from build123d import *

# Parameters (mm, degrees)
F1_W          = 508
F1_H          = 254
F2_DEPTH      = 63.5
F4_R          = 38.1
F5_DEPTH      = 127
F5_DEPTH_BACK = 127
F6_R          = 57.15
F7_DEPTH      = 127
F7_DEPTH_BACK = 127
F3_R          = 19.05
F8_DEPTH      = 127
F9_SIZE2      = 12.7
F9_SIZE       = 12.7


with BuildPart() as f2:
    # F1 (on face) → F2 (new body)
    with BuildSketch(Plane.XY):
        with Locations((0, -127)):
            Rectangle(F1_W, F1_H)
    extrude(amount=F2_DEPTH)

    # F4 (on face) → F5 (cut, two sides)
    with BuildSketch(Plane.XY.offset(63.5)) as f5_sk:
        with Locations((-63.5, -127)):
            Circle(F4_R)
    extrude(amount=F5_DEPTH, mode=Mode.SUBTRACT)
    extrude(f5_sk.sketch, amount=-F5_DEPTH_BACK, mode=Mode.SUBTRACT)

    # F6 (on face) → F7 (cut, two sides)
    with BuildSketch(Plane.XY.offset(63.5)) as f7_sk:
        with Locations((127, -127)):
            Circle(F6_R)
    extrude(amount=F7_DEPTH, mode=Mode.SUBTRACT)
    extrude(f7_sk.sketch, amount=-F7_DEPTH_BACK, mode=Mode.SUBTRACT)

    # F3 (on face) → F8 (cut)
    with BuildSketch(Plane.XY.offset(63.5)):
        with Locations((-190.5, -127)):
            Circle(F3_R)
    extrude(amount=-F8_DEPTH, mode=Mode.SUBTRACT)

    # F9
    f9_edges = [f2.edges().sort_by_distance(p)[0] for p in [
        (-254, -127, 0),
        (0, 0, 0),
        (-254, -254, 31.75),
        (254, -254, 31.75),
        (0, -254, 0),
        (0, -254, 63.5),
        (254, 0, 31.75),
        (254, -127, 0),
        (254, -127, 63.5),
        (0, 0, 63.5),
        (-254, -127, 63.5),
        (-209.55, -127, 63.5),
        (-101.6, -127, 63.5),
        (69.85, -127, 63.5),
        (-209.55, -127, 0),
        (-101.6, -127, 0),
        (69.85, -127, 0),
    ]]
    chamfer(f9_edges, length=F9_SIZE, length2=F9_SIZE2)


solid = f2.part
Here's how the part is built. I have some questions about the finished solid (model axes, mm). Give positions to 0.01 mm unless a question says otherwise; leave off trailing zeros. Order: outer loops, then holes, each group sorted by start corner. A loop starts at its lowest first (then second) coordinate and runs counter-clockwise, first axis right, second up. Notation, with made-up numbers: (10, -4) -> (21, -4) arc R16 cw to (21, 0) -> close; hole circle Ø8 at (85.5, 26.25). An arc over 180 degrees is marked (long way). Use a Markdown table: item, result. Add a question column.
Item 1: Will these pins go through, and if not, where does the flat tip stop? pin 1 (1 mm diameter, centred on x = 33.5, z = 10, fed in from +Y); pin 2 (6 mm diameter, centred on x = 81, y = -89.5, fed in from +Z); pin 3 (8 mm diameter, centred on x = -1.5, y = -108.5, fed in from -Z).
Item 2: Imagine slicing it at C-C on z = 23. Please give me the cut outline in (x, y).
Item 3: Imagine slicing it at D-D on x = -7. Please give me the cut outline in (y, z).
Item 4: If we mould it in two halves opening along Y, with no side actions, what happens to faces 1 (the face through (-45.92, -160.8, 32.02)), 2 (the face through (180.362, -149.125, 12.083)), 3 (the face through (-245.14, -245.31, 55.65)), 4 (the face through (-254, -122, 31))? For each: pulls with the +Y half, pulls with the -Y half, needs draft (parallel to the pull), parting line crosses it, or undercut.
Item 5: I need wall thicknesses on line 1 (Y direction, x = 127, z = 21); line 2 (Y direction, x = -63.5, z = 33); line 3 (X direction, y = -120.5, z = 56). Which ranges of each line are inside material? Lowest first, please.
Item 6: Imagine slicing it at B-B on x = 127. Please give me the cut outline in (y, z), plus the area to 3 significant figures.
Item 7: Imagine slicing it at A-A on y = -127. Give the number of separate pieces and of enclosed holes in the cut face, plus the area to 3 significant figures.
Data:
| question | item | result |
|---|---|---|
| 1 | pin 1 | stops at y = -2.2 |
| 1 | pin 2 | stops at z = 56 |
| 1 | pin 3 | stops at z = 0 |
| 2 | outline | (-254, -241.3) -> (-241.3, -254) -> (241.3, -254) -> (254, -241.3) -> (254, -12.7) -> (241.3, 0) -> (-254, 0) -> close; hole circle Ø38.1 at (-190.5, -127); hole circle Ø76.2 at (-63.5, -127); hole circle Ø114.3 at (127, -127) |
| 3 | outline | (-254, 12.7) -> (-241.3, 0) -> (-12.7, 0) -> (0, 12.7) -> (0, 50.8) -> (-12.7, 63.5) -> (-241.3, 63.5) -> (-254, 50.8) -> close |
| 4 | face 1 | undercut |
| 4 | face 2 | undercut |
| 4 | face 3 | pulls with the -Y half |
| 4 | face 4 | needs draft |
| 5 | line 1 | y = -254 to -184.15, -69.85 to 0 |
| 5 | line 2 | y = -254 to -165.1, -88.9 to 0 |
| 5 | line 3 | x = -248.8 to -213.86, -167.14 to -106.31, -20.69 to 64.99, 189.01 to 248.8 |
| 6 | outline | (-254, 12.7) -> (-241.3, 0) -> (-196.85, 0) -> (-184.15, 12.7) -> (-184.15, 50.8) -> (-196.85, 63.5) -> (-241.3, 63.5) -> (-254, 50.8) -> close; (-69.85, 12.7) -> (-57.15, 0) -> (-12.7, 0) -> (0, 12.7) -> (0, 50.8) -> (-12.7, 63.5) -> (-57.15, 63.5) -> (-69.85, 50.8) -> close |
| 6 | area | 8,230 mm² |
| 7 | separate pieces | 4 |
| 7 | enclosed holes | 0 |
| 7 | area | 16,500 mm² |
